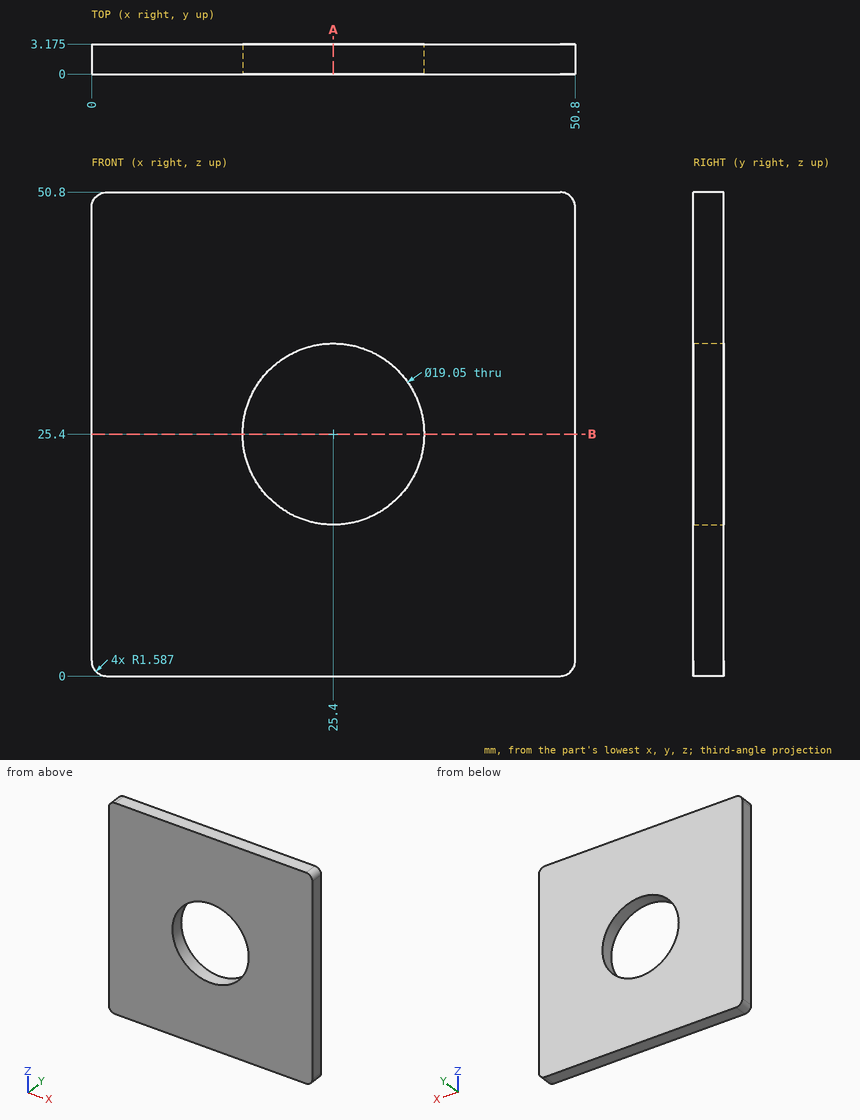
For this review, use the dimensioned drawing (mm, ordinates from the lowest corner) and the shaded views. Give positions to 0.01 mm unless a question says otherwise; leave off trailing zeros. Order: outer loops, then holes, each group sorted by start corner. A loop starts at its lowest first (then second) coordinate and runs counter-clockwise, first axis right, second up. Notation, with made-up numbers: (73.25, -11.5) - (132.25, -11.5) arc R19 ccw to (132.25, -1.5) - close; hole circle Ø4 at (78.5, 60). An arc over 180 degrees is marked (long way). Write item = value, one per line. Start each with the question number.
Q1. We need section B-B on z = 25.4. State the section outline as (x, y) points (1 decimal), plus the area to 3 significant figures.
Q2. We need section A-A on x = 25.4. State the section outline as (y, z) points (1 decimal), plus the area to 3 significant figures.
Q3. To check wall thickness, follow L1, parallel to Z at x = 25.4, y = 0.95 (1 decimal); L2, parallel to Z at x = 32.5, y = 0.4; L3, parallel to X at y = 0.8, z = 22.5. State the ranges of each line that lie inside material, in increasing order. Write a range as from..to.
Working result:
q1.outline = (0, 0) - (15.9, 0) - (15.9, 3.2) - (0, 3.2) - close; (34.9, 0) - (50.8, 0) - (50.8, 3.2) - (34.9, 3.2) - close
q1.area = 101 mm²
q2.outline = (0, 0) - (3.2, 0) - (3.2, 15.9) - (0, 15.9) - close; (0, 34.9) - (3.2, 34.9) - (3.2, 50.8) - (0, 50.8) - close
q2.area = 101 mm²
q3.L1 = 0..15.9, 34.9..50.8
q3.L2 = 0..19.05, 31.75..50.8
q3.L3 = 0..16.33, 34.47..50.8
